Work out the finished part from the listing and answer in its coordinate system (mm). Round coordinates to 2 decimals unless told otherwise and drop trailing zeros. Write each loop counter-clockwise with the first axis right and the second up, starting at its lowest first coordinate (ties: lowest second). Pieces come first, ordered by that corner, then holes. Notation, with made-up numbers: (52.5, 15.5) -> (88.5, 15.5) arc R35 cw to (88.5, 47.5) -> close; hole circle Ø11 at (84.5, -4). An arc over 180 degrees is marked (long way). Answer as a JSON object with one key per item and string values. Group by question number.
from build123d import *

# Parameters (mm, degrees)
SKETCH1_R           = 6.5
BOSS_EXTRUDE1_DEPTH = 10


with BuildPart() as part:
    # Sketch1 → Boss-Extrude1 (new body)
    with BuildSketch(Plane(origin=(0, 0, 0), x_dir=(1, 0, 0), z_dir=(0, 1, 0))):
        with BuildLine():
            Line((16, 88), (16, 50.079936102))
            ThreePointArc((16, 50.079936102), (17.85785805, 41.23153977), (23.117647059, 33.877603834))
            ThreePointArc((23.117647059, 33.877603834), (8.830347529, -42.810505744), (-53.85766764, 3.615842732))
            ThreePointArc((-53.85766764, 3.615842732), (-48.982974202, 10.361725626), (-40.752437215, 9.125670194))
            Line((-40.752437215, 9.125670194), (-16.977471788, -10.742671935))
            ThreePointArc((-16.977471788, -10.742671935), (3.641076169, -7.777232518), (-1.512195122, 12.405981939))
            ThreePointArc((-1.512195122, 12.405981939), (-12.095770915, 22.346620452), (-16, 36.331804249))
            Line((-16, 36.331804249), (-16, 88))
            ThreePointArc((-16, 88), (0, 104), (16, 88))
        make_face()
        with Locations(Location((0, 88, 0), (0, 0, 270))):
            Circle(SKETCH1_R, mode=Mode.SUBTRACT)
    extrude(amount=BOSS_EXTRUDE1_DEPTH)


solid = part.part
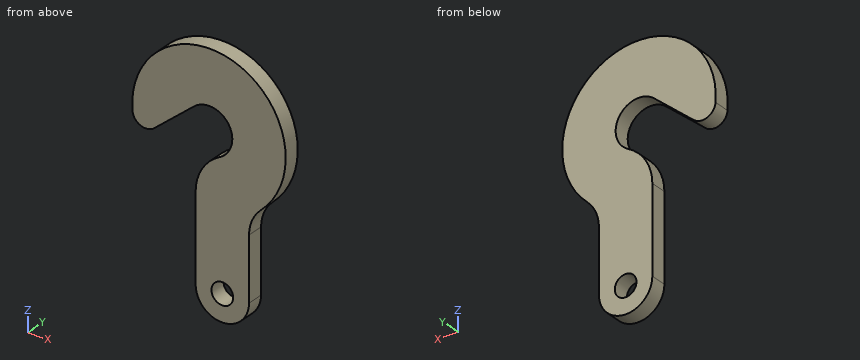
1) A cutting plane is placed at C-C on z = -2. Determine the outline of the cut face in (x, y).
2) A cutting plane is placed at D-D on z = -76. Determine the outline of the cut face in (x, y), plus the area to 3 significant figures.
3) A cutting plane is placed at A-A on y = 1.5. Determine the outline of the cut face in (x, z).
4) A cutting plane is placed at B-B on x = -8. Determine the outline of the cut face in (y, z), plus the area to 3 significant figures.
5) Straight lines are drawn through the part: L1, parallel to Z at x = -2.5, y = 5.75; L2, parallel to X at y = 3.5, z = -66; L3, parallel to Z at x = 1, y = 9.75. For each, find the intervals that lie inside material, in ascending order.
6) Each of these flat-tipped pins is pushed along its axis until it touches: P1, Ø5, axis at y = 8, z = -42, coming from the -X side; P2, Ø4, axis at x = 24, y = 5, coming from the +Z side; P3, Ø2, axis at x = 5, y = 3.5, coming from the +Z side. Where does it stop, or does it pass through?
Established:
{
 "1": {"outline": "(-53.96, 0) -> (-32.23, 0) -> (-32.23, 10) -> (-53.96, 10) -> close; (5.86, 0) -> (37.96, 0) -> (37.96, 10) -> (5.86, 10) -> close"},
 "2": {"outline": "(-16, 0) -> (16, 0) -> (16, 10) -> (-16, 10) -> close", "area": "320 mm²"},
 "3": {"outline": "(-53.86, -3.62) arc R8 ccw to (-40.75, -9.13) -> (-16.98, 10.74) arc R14 cw (long way) to (-1.51, -12.41) arc R27 ccw to (-16, -36.33) -> (-16, -88) arc R16 ccw to (16, -88) -> (16, -50.08) arc R22 cw to (23.12, -33.88) arc R46 ccw (long way) to start; hole circle Ø13 at (0, -88)"},
 "4": {"outline": "(0, -101.86) -> (10, -101.86) -> (10, -17.15) -> (0, -17.15) -> close; (0, 14) -> (10, 14) -> (10, 46) -> (0, 46) -> close", "area": "1,170 mm²"},
 "5": {"L1": "z = -103.8 to -94, -82 to -12.95, 12.87 to 45.67", "L2": "x = -16 to 16", "L3": "z = -103.97 to -94.42, -81.58 to -10.72, 10.72 to 45.11"},
 "6": {"P1": "stops at x = -16", "P2": "stops at z = 34.87", "P3": "stops at z = 44.41"}
}
